Autodesk Inventor part; units mm, degrees
ref_plane "YZ Plane" through (0, 0, 0) normal (1, 0, 0) x (0, 1, 0)
ref_plane "XZ Plane" through (0, 0, 0) normal (0, 1, 0) x (-1, 0, 0)
ref_plane "XY Plane" through (0, 0, 0) normal (0, 0, 1) x (1, 0, 0)
sketch "Sketch1" plane through (0, 0, 0) normal (0, 1, 0) x (-1, 0, 0)
  line L0 (-7.3323, 0) -> (-3.6662, 6.35)
  line L1 (-3.6662, 6.35) -> (3.6662, 6.35)
  line L2 (3.6662, 6.35) -> (7.3323, 0)
  line L3 (7.3323, 0) -> (3.6662, -6.35)
  line L4 (3.6662, -6.35) -> (-3.6662, -6.35)
  line L5 (-3.6662, -6.35) -> (-7.3323, 0)
  circle A0 centre (0, 0) radius 6.875
  circle A1 centre (0, 0) radius 6.35
  line L6 (-2.7496, -4.7625) -> (2.7496, -4.7625)
  line L7 (2.7496, -4.7625) -> (5.4993, 0)
  line L8 (5.4993, 0) -> (2.7496, 4.7625)
  line L9 (2.7496, 4.7625) -> (-2.7496, 4.7625)
  line L10 (-2.7496, 4.7625) -> (-5.4993, 0)
  line L11 (-5.4993, 0) -> (-2.7496, -4.7625)
  circle A2 centre (0, 0) radius 4.7625
  circle A3 centre (0, 0) radius 5.125
  circle A4 centre (0, 0) radius 9.525
  circle A5 centre (0, 0) radius 5.9436
  circle A6 centre (0, 0) radius 2.5527
  circle A7 centre (0, 0) radius 2.0193
  circle A8 centre (0, 0) radius 3.175
  circle A9 centre (0, 0) radius 8.7313
  point P0 (-4.1818, 5.457)
  point P1 (-2.635, 6.35)
  point P2 (-6.8168, -0.893)
  point P3 (-6.8168, 0.893)
  point P4 (-2.635, -6.35)
  point P5 (-4.1818, -5.457)
  point P6 (4.1818, -5.457)
  point P7 (2.635, -6.35)
  point P8 (6.8168, -0.893)
  point P9 (6.8168, 0.893)
  point P10 (2.635, 6.35)
  point P11 (4.1818, 5.457)
  point P12 (3.1778, -4.0208)
  point P13 (1.8932, -4.7625)
  point P14 (5.071, -0.7417)
  point P15 (5.071, 0.7417)
  point P16 (1.8932, 4.7625)
  point P17 (3.1778, 4.0208)
  point P18 (-3.1778, 4.0208)
  point P19 (-1.8932, 4.7625)
  point P20 (-5.071, -0.7417)
  point P21 (-5.071, 0.7417)
  point P22 (-1.8932, -4.7625)
  point P23 (-3.1778, -4.0208)
  dimension "d0" = 12.7
  dimension "d1" = 13.75
  dimension "d2" = 12.7
  dimension "d3" = 9.525
  dimension "d4" = 10.25
  dimension "d5" = 19.05
  dimension "d6" = 11.8872
  dimension "d7" = 5.1054
  dimension "d8" = 4.0386
  dimension "d9" = 6.35
  dimension "d153" = 0.7937
extrude "BaseProfile625Round" add sketch "Sketch1" along normal mid plane 93.218 contours L0 A0 L5 | A0 L0 | L0 A1 L5 A0 | L5 A0 | L0 A0 L1 A1 | A1 | L0 L1 A0 | A1 L4 A0 L5 | A0 L4 L5 | L1 A0 | L1 A0 L2 A1 | A1 L3 A0 L4 | L4 A0 | L1 L2 A0 | L2 A0 | L2 A0 L3 A1 | A0 L3 L4 | L3 A0 | L2 L3 A0 | L11 A3 L6 | A3 L11 A2 L6 | L6 A3 | A3 L11 | A2 L7 A3 L6 | A2 | A3 L7 L6 | L11 A3 L10 A2 | L11 L10 A3 | L7 A3 | A2 L8 A3 L7 | L10 A3 | L10 A3 L9 A2 | A3 L8 L7 | L10 L9 A3 | L9 A3 | L9 A3 L8 A2 | L8 A3 | L9 L8 A3 | A4 | A5 | A6 | A7 | A8 | A9
extrude "BaseProfileRoundTube" [suppressed]
extrude "BaseProfile500Hex" [suppressed]
extrude "BaseProfile500Thunderhex" cut sketch "Sketch1" along normal mid plane 914.4 contours L0 A0 L5 | A0 L0 | L5 A0 | L0 L1 A0 | A0 L4 L5 | L1 A0 | L4 A0 | L1 L2 A0 | L2 A0 | A0 L3 L4 | L3 A0 | L2 L3 A0 | A4 | A9
extrude "BaseProfile500Round" [suppressed]
extrude "BaseProfile375Hex" [suppressed]
extrude "BaseProfile375Thunderhex" [suppressed]
extrude "BaseProfile375Round" [suppressed]
extrude "TopShaftProfile1Hex500" [suppressed]
extrude "TopShaftProfile1ThunderHex500" [suppressed]
extrude "TopShaftProfile1Round500" [suppressed]
extrude "TopShaftProfile1Hex375" [suppressed]
extrude "TopShaftProfile1ThunderHex375" [suppressed]
extrude "TopShaftProfile1Round375" [suppressed]
extrude "TopShaftProfile2ThunderHex500" [suppressed]
extrude "TopShaftProfile2Round500" [suppressed]
extrude "TopShaftProfile2Hex375" [suppressed]
extrude "TopShaftProfile2ThunderHex375" [suppressed]
extrude "TopShaftProfile2Round375" [suppressed]
sketch "Sketch2" plane through (0, 0, 0) normal (1, 0, 0) x (0, 1, 0)
  line L0 (-40.8112, 0) -> (47.9537, 0)
  line L1 (0, -2.6658) -> (0, 15.9951)
  line L2 (53.7515, 4.4704) -> (54.8945, 4.4704)
  line L3 (54.8945, 4.4704) -> (54.8945, 4.7625)
  line L4 (54.8945, 4.7625) -> (55.974, 4.7625)
  line L5 (55.974, 4.7625) -> (56.482, 4.2545)
  line L6 (56.482, 4.2545) -> (56.482, 0)
  line L7 (53.7515, 4.4704) -> (53.7515, 0) construction
  line L8 (53.7515, 4.4704) -> (53.7515, 4.7625)
  line L9 (53.7515, 4.7625) -> (46.609, 4.7625)
  line L10 (46.609, 4.7625) -> (46.609, 0)
  line L11 (46.609, 0) -> (56.482, 0)
  line L12 (-46.609, 5.9436) -> (-47.752, 5.9436)
  line L13 (-47.752, 5.9436) -> (-47.752, 6.35)
  line L14 (-47.752, 6.35) -> (-48.8315, 6.35)
  line L15 (-48.8315, 6.35) -> (-49.3395, 5.842)
  line L16 (-49.3395, 5.842) -> (-49.3395, 0)
  line L17 (-46.609, 5.9436) -> (-46.609, 0) construction
  line L18 (-46.609, 5.9436) -> (-46.609, 6.35)
  line L19 (-46.609, 6.35) -> (-46.609, 6.35)
  line L20 (-46.609, 6.35) -> (-46.609, 0)
  line L21 (-46.609, 0) -> (-49.3395, 0)
  line L22 (0, 0) -> (0, 13.3292)
  line L23 (46.609, 0) -> (46.609, 4.7625)
  point P0 (25.4, 5.9436)
  point P1 (-49.3395, 0)
  point P2 (-46.609, 0)
  point P3 (30.955, 4.7625)
  point P4 (-17.4625, 6.2865)
  point P5 (25.4, 4.7625)
  point P6 (19.4005, 4.7625)
  point P7 (-25.4, 4.7625)
  point P8 (-26.543, 4.7625)
  dimension "TopBearingRoundDia2" = 9.525
  dimension "d65" = 45
  dimension "RetainingRingChamferSize2" = 0.508
  dimension "d72" = 46.609
  dimension "TopSnapRingDia2" = 8.9408
  dimension "d119" = 0.508
  dimension "d120" = 45
  dimension "d135" = 46.609
  dimension "d138" = 56.482
  dimension "d139" = 54.8945
  dimension "d140" = 53.7515
  dimension "d141" = 11.8872
  dimension "d142" = 12.7
  dimension "d143" = 47.752
  dimension "d144" = 46.609
  dimension "d145" = 49.3395
revolve "TopRetentionGroove&BearingRound" [suppressed]
sketch "Sketch3" plane through (0, 46.609, 0) normal (0, 1, 0) x (1, 0, 0)
  point P0 (0, 0)
  point P1 (0, 0)
hole "TopShaftTappedHole" at (0, 46.609, 0) direction (0, -1, 0) diameter 6.35 depth 15.875 tip angle 118
thread "TopShaftThread"
extrude "BottomShaftProfile1Hex500" [suppressed]
extrude "BottomShaftProfile1ThunderHex500" [suppressed]
extrude "BottomShaftProfile1Round500" [suppressed]
extrude "BottomShaftProfile1Hex375" [suppressed]
extrude "BottomShaftProfile1ThunderHex375" [suppressed]
extrude "BottomShaftProfile2ThunderHex500" [suppressed]
extrude "BottomShaftProfile1Round375" [suppressed]
extrude "BottomShaftProfile2Round500" [suppressed]
extrude "BottomShaftProfile2Hex375" [suppressed]
extrude "BottomShaftProfile2ThunderHex375" [suppressed]
extrude "BottomShaftProfile2Round375" [suppressed]
sketch "Sketch4" plane through (0, -46.609, 0) normal (0, -1, 0) x (1, 0, 0)
  point P0 (0, 0)
  point P1 (0, 0)
hole "BottomShaftTappedHole" at (0, -46.609, 0) direction (0, 1, 0) diameter 6.35 depth 15.875 tip angle 118
thread "BottomShaftThread"
revolve "BottomRetentionGroove&BearingRound" [suppressed]
extrude "BaseProfile375ThunderhexHole" [suppressed]
extrude "BaseProfile500ThunderhexHole" cut sketch "Sketch1" along normal mid plane 914.4 contours A6 | A7
equation "\"d18\" = BottomShaftProfile1Depth + TopShaftProfile1Depth + BaseShaftLength + TopShaftProfile2Depth + BottomShaftProfile2Depth"
equation "\"d72\" = 0.5 * d18"
equation "\"BaseShaftLength\" = 93.218"
equation "\"TopShaftProfile1Depth\" = 0"
equation "\"TopShaftProfile2Depth\" = 0"
equation "\"BottomShaftProfile1Depth\" = 0"
equation "\"BottomShaftProfile2Depth\" = 0"
equation "\"TopShaftHoleDia\" = 6.35"
equation "\"BottomShaftHoleDia\" = 6.35"
equation "\"TopBearingRoundDia\" = 9.525"
equation "\"TopGrooveWidth\" = 1.143"
equation "\"TopBearingRoundDistance\" = 7.14248"
equation "\"TopSnapRingDia\" = 8.9408"
equation "\"BottomBearingRoundDia\" = 12.7"
equation "\"BottomGrooveWidth\" = 1.143"
equation "\"BottomBearingRoundDistance\" = 0"
equation "\"BottomSnapRingDia\" = 11.8872"
equation "\"RoundTubeDia\" = 19.05"
properties part number "GreyT Claw 2 Pivot Shaft" material "Aluminum 6061"
Geometry check sheet. Reference: the model listing, model coordinates, mm. A direction names the side the tool comes from. Give positions to 0.01 mm unless a question says otherwise; leave off trailing zeros. Write each loop counter-clockwise with the first axis right and the second up, starting at its lowest first coordinate (ties: lowest second). Pieces come first, ordered by that corner, then holes.
1) Go/stop test with flat-tipped pins: pin 1 Ø1 at (y, z) = (30.5, 2.5) entering from -X; pin 2 Ø8 at (x, y) = (-3.5, -7) entering from +Z; pin 3 Ø1 at (y, z) = (28, 4) entering from -X. Record where each tip stops, or that it passes through.
Values follow:
pin 1: stops at x = -6.18
pin 2: stops at z = 6.35
pin 3: stops at x = -5.31
2) Set-up check for faces 5 (the face through (3.1, -38.56, 0.69)), 6 (the face through (2, 46.609, 3)): record each of +Z, -Z, +X, -X, +Y, -Y from which the full face is reachable in a straight line by a thin tool's end or side.
Values follow:
face 5: -Y
face 6: +Z, -Z, +X, -X, +Y
3) Thickness scan on line 1 (X direction, y = 36.75, z = 0) (3 decimals); line 2 (Z direction, x = 0, y = -38) (3 decimals); line 3 (X direction, y = -5, z = 0) (3 decimals). Record the ranges inside material, lowest first.
Values follow:
line 1: x = -6.875 to -3.175, 3.175 to 6.875
line 2: z = -6.35 to -3.175, 3.175 to 6.35
line 3: x = -6.875 to -2.553, 2.553 to 6.875
4) Cross-section at B-B (y = -34.5). Record the boundary of the cut face in (x, z) (3 decimals), plus the area to 3 significant figures.
Values follow:
outline: (-6.817, -0.893) - (-4.182, -5.457) arc R6.875 ccw to (-2.635, -6.35) - (2.635, -6.35) arc R6.875 ccw to (4.182, -5.457) - (6.817, -0.893) arc R6.875 ccw to (6.817, 0.893) - (4.182, 5.457) arc R6.875 ccw to (2.635, 6.35) - (-2.635, 6.35) arc R6.875 ccw to (-4.182, 5.457) - (-6.817, 0.893) arc R6.875 ccw to start; hole circle Ø6.35 at (0, 0)
area: 106 mm2
5) Cross-section at D-D (y = -6). Record the boundary of the cut face in (x, z) (3 decimals), plus the area to 3 significant figures.
Values follow:
outline: (-6.817, -0.893) - (-4.182, -5.457) arc R6.875 ccw to (-2.635, -6.35) - (2.635, -6.35) arc R6.875 ccw to (4.182, -5.457) - (6.817, -0.893) arc R6.875 ccw to (6.817, 0.893) - (4.182, 5.457) arc R6.875 ccw to (2.635, 6.35) - (-2.635, 6.35) arc R6.875 ccw to (-4.182, 5.457) - (-6.817, 0.893) arc R6.875 ccw to start; hole circle Ø5.105 at (0, 0)
area: 117 mm2
6) Cross-section at C-C (x = 0). Record the boundary of the cut face in (y, z) (3 decimals).
Values follow:
outline: (-46.609, -6.35) - (46.609, -6.35) - (46.609, -3.175) - (30.734, -3.175) - (30.36, -2.553) - (-30.36, -2.553) - (-30.734, -3.175) - (-46.609, -3.175) - close; (-46.609, 3.175) - (-30.734, 3.175) - (-30.36, 2.553) - (30.36, 2.553) - (30.734, 3.175) - (46.609, 3.175) - (46.609, 6.35) - (-46.609, 6.35) - close
7) Cross-section at A-A (z = 0). Record the boundary of the cut face in (x, y) (3 decimals), plus the area to 3 significant figures.
Values follow:
outline: (-6.875, -46.609) - (-3.175, -46.609) - (-3.175, -30.734) - (-2.553, -30.36) - (-2.553, 30.36) - (-3.175, 30.734) - (-3.175, 46.609) - (-6.875, 46.609) - close; (2.553, -30.36) - (3.175, -30.734) - (3.175, -46.609) - (6.875, -46.609) - (6.875, 46.609) - (3.175, 46.609) - (3.175, 30.734) - (2.553, 30.36) - close
area: 766 mm2
8) Release check for a two-part mould opening along X. For faces 1 (the face through (3.1, 38.56, -0.69)), 2 (the face through (-3.448, -0.653, -5.948)), 3 (the face through (6.875, -0.653, -0.013)), 4 (the face through (-2.435, 0.425, 0.767)) record: released by +X, released by -X, zero draft, split by the parting line, or undercut.
Values follow:
face 1: undercut
face 2: released by -X
face 3: released by +X
face 4: undercut
